Autodesk Inventor part; units mm, degrees
ref_plane "YZ Plane" through (0, 0, 0) normal (1, 0, 0) x (0, 1, 0)
ref_plane "XZ Plane" through (0, 0, 0) normal (0, 1, 0) x (-1, 0, 0)
ref_plane "XY Plane" through (0, 0, 0) normal (0, 0, 1) x (1, 0, 0)
sketch "Sketch1" plane through (0, 0, 0) normal (0, 0, 1) x (1, 0, 0)
  circle A0 centre (0, 0) radius 2.0828
  dimension "d0" = 4.1656
extrude "Extrusion1" add sketch "Sketch1" along normal blind 19.05
sketch "Sketch2" plane through (0, 0, 0) normal (0, 1, 0) x (-1, 0, 0)
  line L0 (0, 0) -> (0, -2.2098)
  line L1 (0, 0) -> (3.9624, 0)
  line L2 (0, -2.2098) -> (2.032, -2.2098)
  line L3 (3.9624, 0) -> (3.9624, 3.6562) construction
  arc A0 (2.032, -2.2098) -> (3.9624, -0.4599) centre (0.1837, 1.7689) ccw
  line L4 (4.5847, 0.6553) -> (4.5847, -0.2608) construction
  line L5 (3.9624, -0.4599) -> (3.9624, 0)
  dimension "d3" = 2.2098
  dimension "d6" = 2.032
  dimension "d19" = 3.9624
revolve "Revolution1" add sketch "Sketch2" angle 360 about axis through (0, 0, 0) along (0, 0, -1)
sketch "Sketch3" plane through (0, 0, -2.2098) normal (0, 0, -1) x (-1, 0, 0)
  circle A0 centre (0, 0) radius 2.032
  line L0 (-0.6874, 1.1906) -> (0.6874, 1.1906)
  line L1 (0.6874, 1.1906) -> (1.3748, 0)
  line L2 (1.3748, 0) -> (0.6874, -1.1906)
  line L3 (0.6874, -1.1906) -> (-0.6874, -1.1906)
  line L4 (-0.6874, -1.1906) -> (-1.3748, 0)
  line L5 (-1.3748, 0) -> (-0.6874, 1.1906)
  dimension "d8" = 2.3813
extrude "Extrusion2" cut sketch "Sketch3" against normal blind 1.5875 contours L0 L1 L2 L3 L4 L5
chamfer "Chamfer1" distance 0.508 angle 45 1 edges at (-2.0828, 0, 19.05)
thread "Thread1"
properties part number "8-32 BHCS x750" material "Steel"
Input: part model. Units: mm. Frame: model coordinates. A direction names the side the tool comes from. Round coordinates to 2 decimals unless told otherwise and drop trailing zeros. Write each loop counter-clockwise with the first axis right and the second up, starting at its lowest first coordinate (ties: lowest second). Pieces come first, ordered by that corner, then holes.
1) Contact query for flat-ended pins moving along their axis: P1, Ø1.5, axis at x = 0, z = -2, coming from the -Y side; P2, Ø4, axis at y = -0.5, z = 14, coming from the -X side; P3, Ø1.2, axis at x = 0.5, y = 0, coming from the -Z side. Output: stop coordinate, or through.
2) Ray query, L1, parallel to Z at x = 0.25, y = 1; L2, parallel to Y at x = 0.25, z = 16.75; L3, parallel to X at y = -1.75, z = -1. Return the intervals inside material, ascending.
3) Draft query along Y for faces 4 (the cylindrical face through (0.52, -3.93, -0.23)), 5 (the flat face through (-1, -1, -2.21)), 6 (the flat face through (0, 0, -0.622)), 7 (the flat face through (1.036, 0.587, -1.427)). Return one class per face: pulls with the +Y half, pulls with the -Y half, needs draft (parallel to the pull), parting line crosses it, or undercut.
4) Cut plane A-A (z = 17.5). Return the cut outline in (x, y), then the cut area to 3 significant figures.
5) Reachability of faces 1 (the flat face through (-1.036, -0.587, -1.427)), 2 (the cylindrical face through (1.987, -0.626, 9.141)), 3 (the flat face through (0, 0, 19.05)) from +Z, -Z, +X, -X, +Y, -Y: full face, straight path, thin tool, end or side. Return the list, or none.
Geometry says:
1. P1: stops at y = -3.37
1. P2: stops at x = -2.08
1. P3: stops at z = -0.62
2. L1: z = -0.62 to 19.05
2. L2: y = -2.07 to 2.07
2. L3: x = -3.13 to 3.13
3. face 4: parting line crosses it
3. face 5: needs draft
3. face 6: undercut
3. face 7: undercut
4. outline: circle Ø4.17 at (0, 0)
4. area: 13.6 mm2
5. face 1: -Z
5. face 2: +Z
5. face 3: +Z, +X, -X, +Y, -Y
